from build123d import *

# Parameters (mm, degrees)
SKETCH1_R                       = 40
SKETCH1_R_2                     = 35
BOSS_EXTRUDE1_DEPTH             = 27
F_3_0MM_DOWEL_HOLE1_D           = 3
F_3_0MM_DOWEL_HOLE1_CSINK_D     = 3.05
F_3_0MM_DOWEL_HOLE1_CSINK_ANGLE = 90


with BuildPart() as part:
    # Sketch1 → Boss-Extrude1 (new body)
    with BuildSketch(Plane.XY):
        Circle(SKETCH1_R)
        Circle(SKETCH1_R_2, mode=Mode.SUBTRACT)
    extrude(amount=BOSS_EXTRUDE1_DEPTH)

    # Ø3.0mm Dowel Hole1 (through all)
    with Locations(Plane(origin=(0, 0, 0), x_dir=(-1, 0, 0), z_dir=(0, 0, -1))):
        with Locations((0, 37), (26.162950904, 26.162950904), (37, 0), (-26.162950904, 26.162950904), (-37, 0), (-26.162950904, -26.162950904), (0, -37), (26.162950904, -26.162950904)):
            CounterSinkHole(F_3_0MM_DOWEL_HOLE1_D / 2, F_3_0MM_DOWEL_HOLE1_CSINK_D / 2, counter_sink_angle=F_3_0MM_DOWEL_HOLE1_CSINK_ANGLE)


solid = part.part
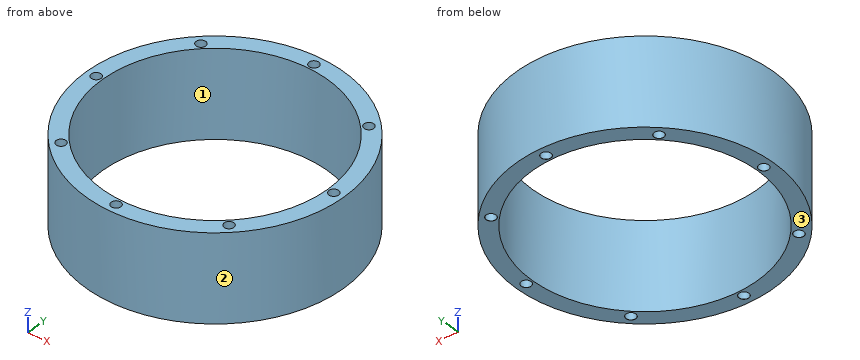
Design review of the part built by this model. Coordinates are the model's own, in mm. Face numbers are marked on the shaded views. Round coordinates to 2 decimals unless told otherwise and drop trailing zeros. Write each loop counter-clockwise with the first axis right and the second up, starting at its lowest first coordinate (ties: lowest second). Pieces come first, ordered by that corner, then holes. Notation, with made-up numbers: (0, 34) -> (43, 34) arc R14 ccw to (43, 47) -> close; hole circle Ø11 at (54.25, -13.5). An arc over 180 degrees is marked (long way). One line per item, written item: value. Start each with the question number.
Q1. Add section A-A (y = 0). Give the boundary of the cut face in (x, z) (3 decimals), then the cut area to 3 significant figures.
Q2. Insertion check: P1, Ø5, axis at x = 30, z = 4, coming from the -Y side; P2, Ø12, axis at y = -15.5, z = 11.5, coming from the -X side; P3, Ø5, axis at x = 20.5, z = 21, coming from the -Y side. Each pin has a flat end and moves straight along its axis. Give the tip position at first contact, or say it passes through.
Q3. The part is to be moulded in two halves that separate along Y. For the marked faces 1, 2 and 3, say which applies: pulls with the +Y half, pulls with the -Y half, needs draft (parallel to the pull), parting line crosses it, or undercut.
Q4. To check wall thickness, follow probe 1 along Y at (x, z) = (26, 21.5); probe 2 along X at (y, z) = (-27.5, 20.25); probe 3 along X at (y, z) = (-25.5, 19). State the ranges of each line that lie inside material, in increasing order.
Q5. Add section D-D (y = 37). Give the boundary of the cut face in (x, z) (3 decimals), then the cut area to 3 significant figures.
Q6. Add section C-C (x = 16). Give the boundary of the cut face in (y, z), then the cut area to 3 significant figures.
Response:
1. outline: (-40, 0) -> (-38.525, 0) -> (-38.5, 0.025) -> (-38.5, 27) -> (-40, 27) -> close; (-35.5, 0.025) -> (-35.475, 0) -> (-35, 0) -> (-35, 27) -> (-35.5, 27) -> close; (35, 0) -> (35.475, 0) -> (35.5, 0.025) -> (35.5, 27) -> (35, 27) -> close; (38.5, 0.025) -> (38.525, 0) -> (40, 0) -> (40, 27) -> (38.5, 27) -> close
1. area: 108 mm^2
2. P1: stops at y = -29.05
2. P2: stops at x = -38.86
2. P3: stops at y = -35.72
3. face 1: undercut
3. face 2: parting line crosses it
3. face 3: needs draft
4. probe 1: y = -30.4 to -27.65, -24.67 to -23.43, 23.43 to 24.67, 27.65 to 30.4
4. probe 2: x = -29.05 to -26.84, -25.48 to -21.65, 21.65 to 25.48, 26.84 to 29.05
4. probe 3: x = -30.82 to -27.51, -24.82 to -23.97, 23.97 to 24.82, 27.51 to 30.82
5. outline: (-15.199, 0) -> (-1.525, 0) -> (-1.5, 0.025) -> (-1.5, 27) -> (-15.199, 27) -> close; (1.5, 0.025) -> (1.525, 0) -> (15.199, 0) -> (15.199, 27) -> (1.5, 27) -> close
5. area: 740 mm^2
6. outline: (-36.66, 0) -> (-31.13, 0) -> (-31.13, 27) -> (-36.66, 27) -> close; (31.13, 0) -> (36.66, 0) -> (36.66, 27) -> (31.13, 27) -> close
6. area: 299 mm^2
